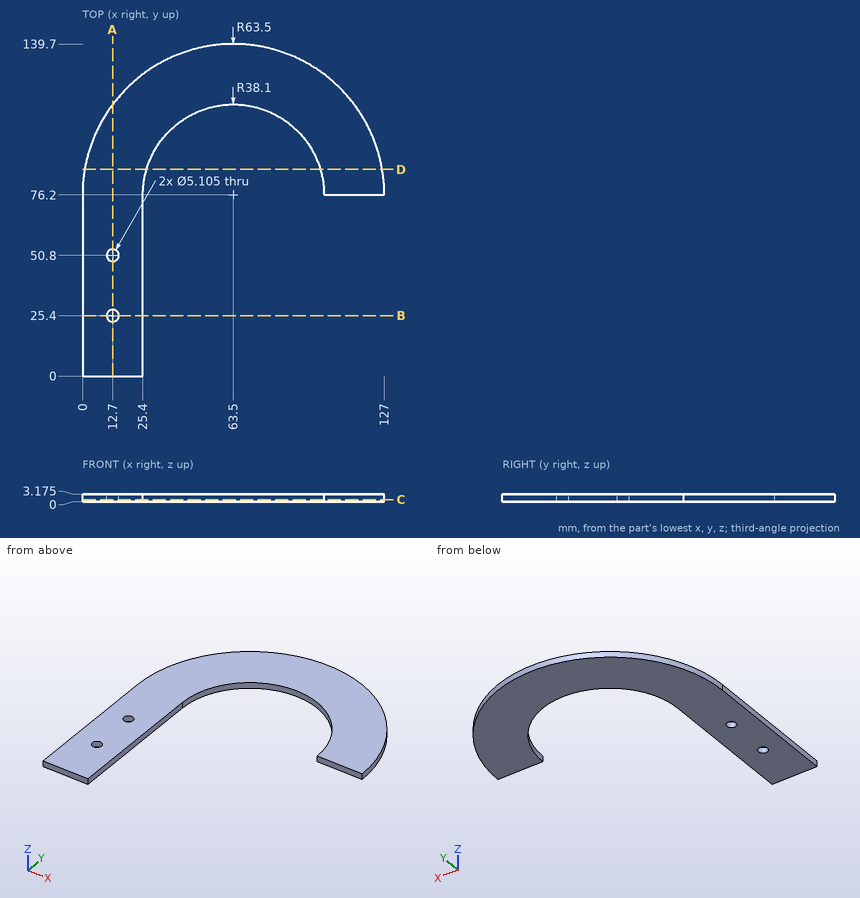
Job drawing, mm, ordinate dimensions from the low corner. One solid piece. Give positions to 0.01 mm unless a question says otherwise; leave off trailing zeros. Write each loop counter-clockwise with the first axis right and the second up, starting at its lowest first coordinate (ties: lowest second). Pieces come first, ordered by that corner, then holes. Notation, with made-up numbers: M 42.5,-28 L 48.5,-28 A15 ccw 48.5,-6 Z; hole C -21,50.5 d5. An arc over 180 degrees is marked long. One line per item, written item: value. Start each with the question number.
Q1. Saw through at D-D, the plane y = 87. Write the cut outline in (x, z) (1 decimal), plus the area to 3 significant figures.
Q2. Saw through at C-C, the plane z = 0.8. Write the cut outline in (x, y) (1 decimal), plus the area to 3 significant figures.
Q3. Probe probe 1 along X at (y, z) = (25.5, 2.5); probe 2 along X at (y, z) = (47, 1); probe 3 along X at (y, z) = (51.5, 1.95) (1 decimal). List the from-to ranges inside material, lowest first. Write a range as [from, to].
Q4. Saw through at A-A, the plane x = 12.7. Write the cut outline in (y, z) (1 decimal).
Q5. Saw through at B-B, the plane y = 25.4. Write the cut outline in (x, z) (1 decimal).
Q6. Drop flat-ended pins along their axis: pin 1 Ø1.6 at (x, z) = (109, 1) entering from -Y; pin 2 Ø4 at (x, y) = (12.7, 25.4) entering from -Z; pin 3 Ø1.5 at (x, z) = (22.5, 1) entering from +Y (1 decimal); pin 4 Ø1 at (y, z) = (20, 1.5) entering from +X. Give the stop position or say it passes through.
Output values:
1. outline: M 0.9,0 L 27,0 L 27,3.2 L 0.9,3.2 Z; M 100,0 L 126.1,0 L 126.1,3.2 L 100,3.2 Z
1. area: 165 mm²
2. outline: M 0,0 L 25.4,0 L 25.4,76.2 A38.1 cw 101.6,76.2 L 127,76.2 A63.5 ccw 0,76.2 Z; hole C 12.7,25.4 d5.1; hole C 12.7,50.8 d5.1
2. area: 5,950 mm²
3. probe 1: x = [0, 10.15], [15.25, 25.4]
3. probe 2: x = [0, 25.4]
3. probe 3: x = [0, 10.2], [15.2, 25.4]
4. outline: M 0,0 L 22.8,0 L 22.8,3.2 L 0,3.2 Z; M 28,0 L 48.2,0 L 48.2,3.2 L 28,3.2 Z; M 53.4,0 L 114.3,0 L 114.3,3.2 L 53.4,3.2 Z
5. outline: M 0,0 L 10.1,0 L 10.1,3.2 L 0,3.2 Z; M 15.3,0 L 25.4,0 L 25.4,3.2 L 15.3,3.2 Z
6. pin 1: stops at y = 76.2
6. pin 2: passes through
6. pin 3: stops at y = 125.3
6. pin 4: stops at x = 25.4
